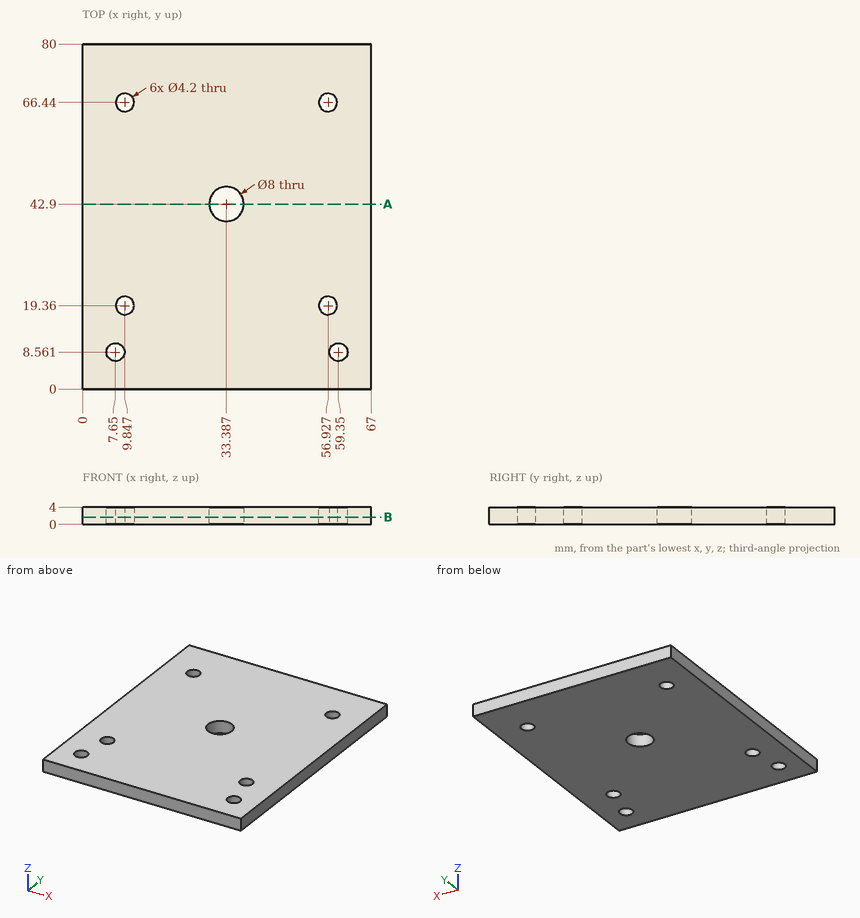
Here's the drawing with two shaded views (mm, measured from the low corner). I have some questions. Coordinates: 2 decimals unless noted, no trailing zeros. Loops run counter-clockwise (first coordinate to the right, second up) from the corner with the lowest first, then second, coordinate; pieces in that order, holes last. Notation, with made-up numbers: M 37.5,34.5 L 88.5,34.5 A12 cw 88.5,41.5 Z; hole C 5,-19.75 d2. An arc over 180 degrees is marked long. Return JSON: item names as keys, results as strings. Group by question number.
Item 1: Imagine slicing it at B-B (z = 1.65). Please give me the cut outline in (x, y), and give its area (3 significant figures).
Item 2: Imagine slicing it at A-A (y = 42.9). Please give me the cut outline in (x, z).
Item 3: If I drill on L1, parallel to Y at x = 57, z = 1.9; L2, parallel to X at y = 44.5, z = 3.4; L3, parallel to Y at x = 6.5, z = 0.9 (1 decimal), over which ranges is the centre line in solid material (lowest first)? Write a range as from..to.
Verdict:
{
 "1": {"outline": "M 0,0 L 67,0 L 67,80 L 0,80 Z; hole C 7.65,8.56 d4.2; hole C 9.85,19.36 d4.2; hole C 9.85,66.44 d4.2; hole C 33.39,42.9 d8; hole C 56.93,19.36 d4.2; hole C 56.93,66.44 d4.2; hole C 59.35,8.56 d4.2", "area": "5,230 mm^2"},
 "2": {"outline": "M 0,0 L 29.39,0 L 29.39,4 L 0,4 Z; M 37.39,0 L 67,0 L 67,4 L 37.39,4 Z"},
 "3": {"L1": "y = 0..17.26, 21.46..64.34, 68.54..80", "L2": "x = 0..29.72, 37.05..67", "L3": "y = 0..6.8, 10.3..80"}
}
